from build123d import *

# Parameters (mm, degrees)
SKETCH_1_W      = 67
SKETCH_1_H      = 10
SKETCH_1_R      = 1.025
SKETCH_1_R_2    = 2.55
EXTRUDE_1_DEPTH = 4.5
FILLET_1_R      = 5


with BuildPart() as part:
    # 草图1 → 凸台-拉伸1 (new body)
    with BuildSketch(Plane.XY):
        with Locations((33.5, -5)):
            Rectangle(SKETCH_1_W, SKETCH_1_H)
        with Locations((5, -5)):
            Circle(SKETCH_1_R, mode=Mode.SUBTRACT)
        with Locations((55, -5)):
            Circle(SKETCH_1_R_2, mode=Mode.SUBTRACT)
    extrude(amount=EXTRUDE_1_DEPTH)

    # 圆角1
    fillet_1_edges = [part.edges().sort_by_distance(p)[0] for p in [
        (0, -10, 2.25),
        (67, -10, 2.25),
        (67, 0, 2.25),
        (0, 0, 2.25),
    ]]
    fillet(fillet_1_edges, radius=FILLET_1_R - 0.0001)  # a hair under: the kernel refuses the full size


solid = part.part
Could you check a few things on this model? Use its own coordinates, in mm. Give positions to 0.01 mm unless a question says otherwise; leave off trailing zeros. Order: outer loops, then holes, each group sorted by start corner. A loop starts at its lowest first (then second) coordinate and runs counter-clockwise, first axis right, second up. Notation, with made-up numbers: (30, -34) - (42, -34) arc R18 cw to (42, -28) - close; hole circle Ø11 at (12, 7.25). An arc over 180 degrees is marked (long way). One line per item, written item: value. Start each with the question number.
1. Imagine slicing it at D-D on y = -8.5. List the corners of the cut face in (x, z) for me.
2. Imagine slicing it at C-C on y = -3.25. List the corners of the cut face in (x, z) for me.
3. For P1, Ø2, axis at y = -7.5, z = 3.5, coming from the +X side, with a flat end and sliding along its axis, tell me the tip position at first contact or that it passes through.
4. Thinking about a two-plate mould opening in X: for faces 1 (the face through (3.976, -4.955, 2.218)), 2 (the face through (65, -1, 2)), 3 (the face through (33, -5, 0)), 4 (the face through (52.452, -4.888, 2.218)), which applies, +X half, -X half, draft (parallel to the pull), parting line (faces both ways), or undercut?
5. Imagine slicing it at B-B on z = 0.8. Give the number of separate pieces and of enclosed holes in the cut face, plus the area to 3 significant figures.
6. If I drill on probe 1 along Y at (x, z) = (55, 3); probe 2 along Y at (x, z) = (5, 2.45) (3 decimals); probe 3 along X at (y, z) = (-4.5, 0.95), over which ranges is the centre line in solid material (lowest first)?
7. Imagine slicing it at A-A on x = 55. List the corners of the cut face in (y, z) for me.
Values:
1. outline: (1.43, 0) - (65.57, 0) - (65.57, 4.5) - (1.43, 4.5) - close
2. outline: (0.32, 0) - (53.15, 0) - (53.15, 4.5) - (0.32, 4.5) - close; (56.85, 0) - (66.68, 0) - (66.68, 4.5) - (56.85, 4.5) - close
3. P1: x = 66.77
4. face 1: undercut
4. face 2: +X half
4. face 3: draft
4. face 4: undercut
5. separate pieces: 1
5. enclosed holes: 2
5. area: 625 mm²
6. probe 1: -10 to -7.55, -2.45 to 0
6. probe 2: -10 to -6.025, -3.975 to 0
6. probe 3: 0.03 to 4.11, 5.89 to 52.5, 57.5 to 66.97
7. outline: (-10, 0) - (-7.55, 0) - (-7.55, 4.5) - (-10, 4.5) - close; (-2.45, 0) - (0, 0) - (0, 4.5) - (-2.45, 4.5) - close
